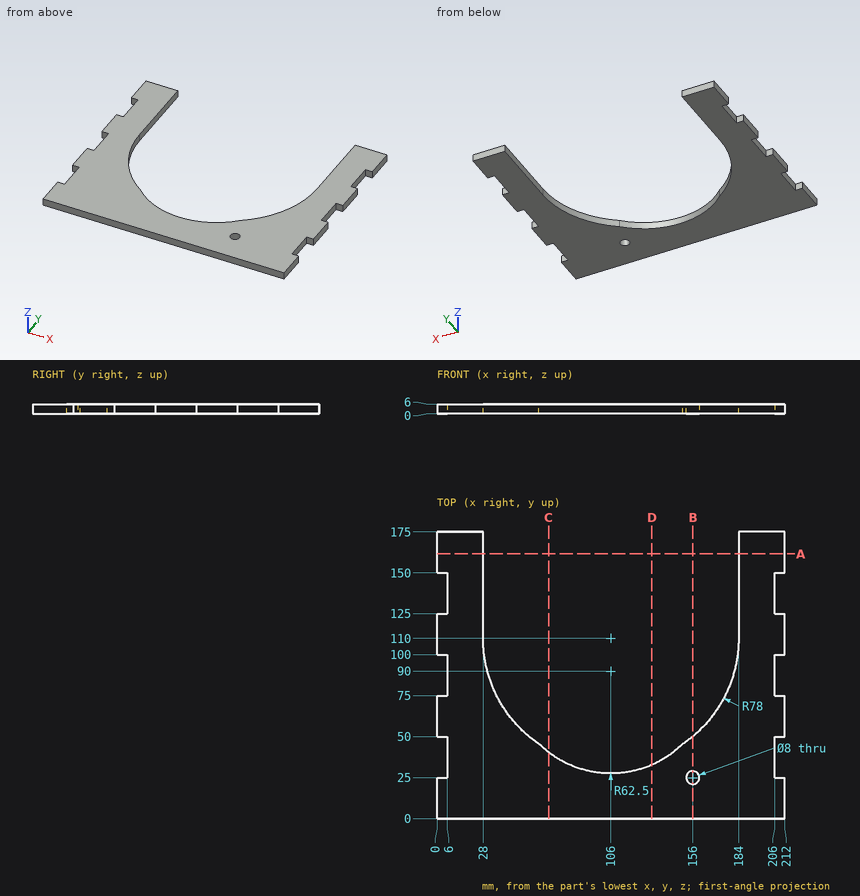
Part print with two shaded views. Sizes in mm from the minimum x, y, z corner. Give positions to 0.01 mm unless a question says otherwise; leave off trailing zeros. Order: outer loops, then holes, each group sorted by start corner. A loop starts at its lowest first (then second) coordinate and runs counter-clockwise, first axis right, second up.
1) Saw through at C-C, the plane x = 68. Write the cut outline in (y, z), then the cut area to 3 significant figures.
2) Pin check, flat tips, straight feed: pin 1 (1.8 mm diameter, centred on y = 41, z = 4.5, fed in from +X); pin 2 (1 mm diameter, centred on x = 175, z = 3, fed in from +Y); pin 3 (3 mm diameter, centred on y = 138, z = 3, fed in from -X). Stop position of each tip, or through.
3) Saw through at A-A, the plane y = 161.5. Write the cut outline in (x, z).
4) Wall check: probe 1 along X at (y, z) = (141, 3.15); probe 2 along Y at (x, z) = (156, 2.1); probe 3 along X at (y, z) = (98, 0.3). Give the ranges that are in metal, low to high.
5) Saw through at D-D, the plane x = 131. Write the cut outline in (y, z).
6) Saw through at B-B, the plane x = 156. Write the cut outline in (y, z), then the cut area to 3 significant figures.
Computed:
1. outline: (0, 0) - (40.38, 0) - (40.38, 6) - (0, 6) - close
1. area: 242 mm2
2. pin 1: stops at x = 206
2. pin 2: stops at y = 74.59
2. pin 3: stops at x = 6
3. outline: (0, 0) - (28, 0) - (28, 6) - (0, 6) - close; (184, 0) - (212, 0) - (212, 6) - (184, 6) - close
4. probe 1: x = 6 to 28, 184 to 206
4. probe 2: y = 0 to 21, 29 to 50.13
4. probe 3: x = 6 to 28.93, 183.07 to 206
5. outline: (0, 0) - (32.72, 0) - (32.72, 6) - (0, 6) - close
6. outline: (0, 0) - (21, 0) - (21, 6) - (0, 6) - close; (29, 0) - (50.13, 0) - (50.13, 6) - (29, 6) - close
6. area: 253 mm2
